Autodesk Inventor part; units mm, degrees
ref_plane "YZ Plane" through (0, 0, 0) normal (1, 0, 0) x (0, 1, 0)
ref_plane "XZ Plane" through (0, 0, 0) normal (0, 1, 0) x (-1, 0, 0)
ref_plane "XY Plane" through (0, 0, 0) normal (0, 0, 1) x (1, 0, 0)
sketch "Sketch1" plane through (0, 0, 0) normal (0, 1, 0) x (-1, 0, 0)
  line L0 (0, 0) -> (-100, 0)
  line L1 (-100, 0) -> (-100, -42)
  line L2 (-100, -42) -> (0, -42)
  line L3 (0, -42) -> (0, 0)
  dimension "d0" = 100
  dimension "d1" = 42
extrude "Extrusion1" add sketch "Sketch1" along normal blind 4
sketch "Sketch2" plane through (0, 4, 0) normal (0, 1, 0) x (1, 0, 0)
  line L0 (0, 0) -> (100, 0) construction
  line L1 (100, 0) -> (100, 42) construction
  line L2 (100, 42) -> (0, 42) construction
  line L3 (0, 42) -> (0, 0) construction
  line L4 (4, 38) -> (96, 38) construction
  line L5 (96, 38) -> (96, 4) construction
  line L6 (96, 4) -> (4, 4) construction
  line L7 (4, 4) -> (4, 38) construction
  line L8 (100, 42) -> (0, 42)
  line L9 (4, 42) -> (4, 34)
  line L10 (4, 34) -> (0, 34)
  line L11 (0, 42) -> (0, 0)
  line L12 (0, 34) -> (0, 42)
  line L13 (0, 42) -> (4, 42)
  line L14 (0, 21) -> (100, 21) construction
  line L15 (50, 42) -> (50, 0) construction
  line L16 (0, 0) -> (100, 0) construction
  line L17 (0, 21) -> (0, 25)
  line L18 (4, 25) -> (0, 25)
  line L19 (4, 25) -> (4, 21)
  line L20 (14, 42) -> (14, 38)
  line L21 (14, 38) -> (22, 38)
  line L22 (22, 38) -> (22, 42)
  line L23 (14, 42) -> (22, 42)
  line L24 (30, 42) -> (38, 42)
  line L25 (38, 42) -> (38, 38)
  line L26 (38, 38) -> (30, 38)
  line L27 (30, 38) -> (30, 42)
  line L28 (50, 38) -> (46, 38)
  line L29 (46, 38) -> (46, 42)
  line L30 (46, 42) -> (50, 42)
  line L31 (4, 0) -> (4, 8)
  line L32 (4, 8) -> (0, 8)
  line L33 (0, 8) -> (0, 0)
  line L34 (0, 0) -> (4, 0)
  line L35 (0, 21) -> (0, 17)
  line L36 (4, 17) -> (0, 17)
  line L37 (4, 17) -> (4, 21)
  line L38 (14, 0) -> (14, 4)
  line L39 (14, 4) -> (22, 4)
  line L40 (22, 4) -> (22, 0)
  line L41 (14, 0) -> (22, 0)
  line L42 (30, 0) -> (38, 0)
  line L43 (38, 0) -> (38, 4)
  line L44 (38, 4) -> (30, 4)
  line L45 (30, 4) -> (30, 0)
  line L46 (50, 4) -> (46, 4)
  line L47 (46, 4) -> (46, 0)
  line L48 (46, 0) -> (50, 0)
  line L49 (100, 42) -> (100, 0) construction
  line L50 (96, 4) -> (96, 38) construction
  line L51 (96, 42) -> (96, 34)
  line L52 (96, 34) -> (100, 34)
  line L53 (100, 42) -> (100, 0)
  line L54 (100, 34) -> (100, 42)
  line L55 (100, 42) -> (96, 42)
  line L56 (100, 21) -> (100, 25)
  line L57 (96, 25) -> (100, 25)
  line L58 (96, 25) -> (96, 21)
  line L59 (86, 42) -> (86, 38)
  line L60 (86, 38) -> (78, 38)
  line L61 (78, 38) -> (78, 42)
  line L62 (86, 42) -> (78, 42)
  line L63 (70, 42) -> (62, 42)
  line L64 (62, 42) -> (62, 38)
  line L65 (62, 38) -> (70, 38)
  line L66 (70, 38) -> (70, 42)
  line L67 (50, 38) -> (54, 38)
  line L68 (54, 38) -> (54, 42)
  line L69 (54, 42) -> (50, 42)
  line L70 (70, 4) -> (70, 0)
  line L71 (62, 4) -> (70, 4)
  line L72 (70, 0) -> (62, 0)
  line L73 (62, 0) -> (62, 4)
  line L74 (54, 4) -> (54, 0)
  line L75 (50, 4) -> (54, 4)
  line L76 (54, 0) -> (50, 0)
  line L77 (78, 4) -> (78, 0)
  line L78 (86, 4) -> (78, 4)
  line L79 (86, 0) -> (78, 0)
  line L80 (86, 0) -> (86, 4)
  line L81 (96, 0) -> (96, 8)
  line L82 (100, 0) -> (96, 0)
  line L83 (96, 8) -> (100, 8)
  line L84 (100, 8) -> (100, 0)
  line L85 (96, 17) -> (96, 21)
  line L86 (100, 21) -> (100, 17)
  line L87 (96, 17) -> (100, 17)
  dimension "d4" = 4
  dimension "d5" = 4
  dimension "d7" = 8
  dimension "d8" = 8
  dimension "d10" = 8
  dimension "d11" = 8
  dimension "d13" = 4
  dimension "d14" = 8
extrude "Extrusion2" cut sketch "Sketch2" against normal up to surface (4 mm away)
sketch "Sketch3" plane through (0, 4, 0) normal (0, 1, 0) x (1, 0, 0)
  line L0 (4, 25) -> (4, 17)
  line L1 (96, 0) -> (96, 8)
  line L2 (4, 17) -> (96, 17)
  line L3 (96, 17) -> (96, 9)
  line L4 (96, 9) -> (4, 9)
  line L5 (4, 9) -> (4, 17)
  line L6 (30, 4) -> (38, 4)
  point P0 (0, 0)
  dimension "d17" = 5
  dimension "d18" = 8
extrude "Extrusion3" add sketch "Sketch3" along normal blind 3
properties part number "front" material "PBT Plastic Black"
Check sheet for the modelled part. Datum: model origin and axes. Units: mm. A direction names the side the tool comes from. Coordinates: 2 decimals unless noted, no trailing zeros. Write each loop counter-clockwise with the first axis right and the second up, starting at its lowest first coordinate (ties: lowest second). Pieces come first, ordered by that corner, then holes. Notation, with made-up numbers: M 46.5,71.25 L 69.5,71.25 A18 ccw 69.5,98.25 Z; hole C 38,37.5 d3. An arc over 180 degrees is marked long. Write item = value, one per line. Start each with the question number.
1. Sectioned sample at C-C (z = -16). Record the cut outline in (x, y).
2. Sectioned sample at D-D (y = 5). Record the cut outline in (x, z).
3. Sectioned sample at A-A (z = -3). Record the cut outline in (x, y).
4. Go/stop test with flat-tipped pins: pin 1 (1.2 mm diameter, centred on y = 1.5, z = -38.5, fed in from +X); pin 2 (2 mm diameter, centred on y = 1.5, z = -2, fed in from -X); pin 3 (3 mm diameter, centred on x = 98, y = 1, fed in from +Z). Record where each tip stops, or that it passes through.
5. Sectioned sample at B-B (x = 77). Record the cut outline in (y, z).
6. Thickness scan on probe 1 along Z at (x, y) = (29, 5.25); probe 2 along Z at (x, y) = (81, 1); probe 3 along Y at (x, z) = (26.5, -32). Record the ranges inside material, lowest first.
7. Tool access check on faces 1 (the flat face through (98, 2, -8)), 2 (the flat face through (46, 2, -2)), 3 (the flat face through (98, 2, -34)), 4 (the flat face through (70, 2, -40)), 5 (the flat face through (51, 5, -9)). Record the directions out of +Z, -Z, +X, -X, +Y, -Y that give a thin tool (end or side, any length) a straight path to the whole face; none if there is none.
The answers:
q1.outline = M 0,0 L 100,0 L 100,4 L 96,4 L 96,7 L 4,7 L 4,4 L 0,4 Z
q2.outline = M 4,-17 L 96,-17 L 96,-9 L 4,-9 Z
q3.outline = M 4,0 L 14,0 L 14,4 L 4,4 Z; M 22,0 L 30,0 L 30,4 L 22,4 Z; M 38,0 L 46,0 L 46,4 L 38,4 Z; M 54,0 L 62,0 L 62,4 L 54,4 Z; M 70,0 L 78,0 L 78,4 L 70,4 Z; M 86,0 L 96,0 L 96,4 L 86,4 Z
q4.pin_1 = 96
q4.pin_2 = 4
q4.pin_3 = -8
q5.outline = M 0,-42 L 4,-42 L 4,-17 L 7,-17 L 7,-9 L 4,-9 L 4,0 L 0,0 Z
q6.probe_1 = -17 to -9
q6.probe_2 = -38 to -4
q6.probe_3 = 0 to 4
q7.face_1 = +Z, +X, +Y, -Y
q7.face_2 = +Z, +Y, -Y
q7.face_3 = -Z, +X, +Y, -Y
q7.face_4 = -Z, +Y, -Y
q7.face_5 = +Z, +X, -X, +Y
